Read the model definition and answer for the solid it produces. Units are mm, in the model's axes. Face numbers are marked on the shaded views. Round coordinates to 2 decimals unless told otherwise and drop trailing zeros. Order: outer loops, then holes, each group sorted by start corner. A loop starts at its lowest first (then second) coordinate and runs counter-clockwise, first axis right, second up. Notation, with made-up numbers: (3.5, 70) - (46.5, 70) arc R21 ccw to (46.5, 89) - close; hole circle Ø11 at (31, -35). An arc over 180 degrees is marked (long way). One line per question, with ' | ' between items. Start each with the question number.
1) The mould has two halves that part along Y. Classify the marked faces 1, 2 and 3: pulls with the +Y half, pulls with the -Y half, needs draft (parallel to the pull), parting line crosses it, or undercut.
2) The part is cut by section C-C, the plane z = 10.25. Give the vertices of the cut face in (x, y).
3) The part is cut by section A-A, the plane x = 0. Give the vertices of the cut face in (y, z), plus the area to 3 significant figures.
4) Straight lines are drawn through the part: line 1 (Y direction, x = 0, z = 6.5); line 2 (Z direction, x = 1.5, y = 0.25); line 3 (X direction, y = 2, z = 7.25). For each, find the intervals that lie inside material, in ascending order. Write a range as from..to.
5) Flat-ended cylindrical pins translate along their axes: pin 1 (6 mm diameter, centred on x = 3.5, z = 12.5, fed in from -Y); pin 2 (4.5 mm diameter, centred on x = 0, y = 0, fed in from -Z); pin 3 (1.5 mm diameter, centred on y = -0.5, z = 14.5, fed in from +X). Find the tip coordinate at first contact, or state that the pin passes through.
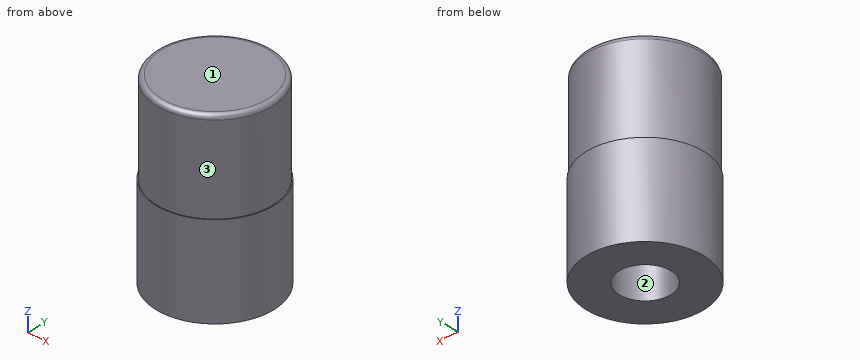
from build123d import *

# Parameters (mm, degrees)
SKETCH1_R           = 6.35
SKETCH1_R_2         = 2.8
BOSS_EXTRUDE2_DEPTH = 10
SKETCH2_R           = 6.35
BOSS_EXTRUDE3_DEPTH = 10
CUT_EXTRUDE1_START  = -10
SKETCH3_R           = 6.35
SKETCH3_R_2         = 6.25
CUT_EXTRUDE1_DEPTH  = 10
FILLET1_R           = 0.5


with BuildPart() as part:
    # Sketch1 → Boss-Extrude2 (new body)
    with BuildSketch(Plane.XY):
        Circle(SKETCH1_R)
        Circle(SKETCH1_R_2, mode=Mode.SUBTRACT)
    extrude(amount=BOSS_EXTRUDE2_DEPTH)

    # Sketch2 → Boss-Extrude3 (add)
    with BuildSketch(Plane.XY.offset(10)):
        Circle(SKETCH2_R)
    extrude(amount=BOSS_EXTRUDE3_DEPTH)

    # Sketch3 → Cut-Extrude1 (cut)
    with BuildSketch(Plane.XY.offset(20).offset(CUT_EXTRUDE1_START)):
        Circle(SKETCH3_R)
        Circle(SKETCH3_R_2, mode=Mode.SUBTRACT)
    extrude(amount=CUT_EXTRUDE1_DEPTH, mode=Mode.SUBTRACT)

    # Fillet1
    fillet1_edges = [part.edges().sort_by_distance(p)[0] for p in [
        (-6.25, 0, 20),
    ]]
    fillet(fillet1_edges, radius=FILLET1_R)


solid = part.part
Values:
1) face 1: needs draft | face 2: undercut | face 3: parting line crosses it
2) outline: circle Ø12.5 at (0, 0)
3) outline: (-6.35, 0) - (-2.8, 0) - (-2.8, 10) - (2.8, 10) - (2.8, 0) - (6.35, 0) - (6.35, 10) - (6.25, 10) - (6.25, 19.5) arc R0.5 ccw to (5.75, 20) - (-5.75, 20) arc R0.5 ccw to (-6.25, 19.5) - (-6.25, 10) - (-6.35, 10) - close | area: 196 mm^2
4) line 1: y = -6.35..-2.8, 2.8..6.35 | line 2: z = 10..20 | line 3: x = -6.03..-1.96, 1.96..6.03
5) pin 1: stops at y = -6.23 | pin 2: stops at z = 10 | pin 3: stops at x = 6.25
